```python
from build123d import *

# Parameters (mm, degrees)
SKETCH1_W           = 3
SKETCH1_H           = 7
BOSS_EXTRUDE1_DEPTH = 3


with BuildPart() as part:
    # Sketch1 → Boss-Extrude1 (new body)
    with BuildSketch(Plane(origin=(0, 0, 0), x_dir=(1, 0, 0), z_dir=(0, 1, 0))):
        Polygon((0, 35), (0, 28), (0, 21), (0, 14), (0, 7), (0, 0), (33, 0), (33, 7), (33, 14), (33, 21), (33, 28), (33, 35), (33, 42), (28.5, 42), (28.5, 39), (21.5, 39), (21.5, 42), (11.5, 42), (11.5, 39), (4.5, 39), (4.5, 42), (0, 42), align=None)
        with Locations((-1.5, 38.5)):
            Rectangle(SKETCH1_W, SKETCH1_H)
        with Locations((-1.5, 24.5)):
            Rectangle(SKETCH1_W, SKETCH1_H)
        with Locations((-1.5, 10.5)):
            Rectangle(SKETCH1_W, SKETCH1_H)
        with Locations((34.5, 10.5)):
            Rectangle(SKETCH1_W, SKETCH1_H)
        with Locations((34.5, 24.5)):
            Rectangle(SKETCH1_W, SKETCH1_H)
        with Locations((34.5, 38.5)):
            Rectangle(SKETCH1_W, SKETCH1_H)
        Polygon((33, 0), (0, 0), (-3, 0), (-3, -1.2), (36, -1.2), (36, 0), align=None)
    extrude(amount=BOSS_EXTRUDE1_DEPTH)


solid = part.part
```
Input: part model. Units: mm. Frame: model coordinates. A direction names the side the tool comes from. Round coordinates to 2 decimals unless told otherwise and drop trailing zeros. Loops run counter-clockwise (first coordinate to the right, second up) from the corner with the lowest first, then second, coordinate; pieces in that order, holes last. Notation, with made-up numbers: M -30,76 L 19,76 A16 cw 19,86 Z; hole C 62.5,80.5 d8. An arc over 180 degrees is marked long. Answer in a Markdown table with one row per item. Add a question column.
1. Section A-A (z = -31). Output: boundary loops of the cut face in (x, y), and give its area (3 significant figures).
2. Contact query for flat-ended pins moving along their axis: pin 1 (5 mm diameter, centred on x = 20, z = -10.5, fed in from -Y); pin 2 (1.5 mm diameter, centred on y = 1.5, z = -2, fed in from +X). Output: stop coordinate, or through.
3. Mould query, pull axis Z, two halves, no side actions, for faces 1 (the face through (16, 1, 1.2)), 2 (the face through (0, 1, -18)), 3 (the face through (28.5, 1, -41)). Classes: released by +Z, released by -Z, zero draft, split by the parting line, or undercut.
4. Set-up query: faces 4 (the face through (36, 1, -38)), 5 (the face through (34, 1, -7)), 6 (the face through (-2, 1, -7)), 7 (the face through (21.5, 1, -40)). Return all of +Z, -Z, +X, -X, +Y, -Y with unobstructed straight access to the full face (end or side cutting, diameter ignored); none if empty.
5. Ray query, probe 1 along Z at (x, y) = (34, 0.3); probe 2 along X at (y, z) = (0.6, -2.5); probe 3 along Z at (x, y) = (6.5, 0.4). Return the intervals inside material, ascending.
Values follow:
| question | item | result |
|---|---|---|
| 1 | outline | M 0,0 L 33,0 L 33,3 L 0,3 Z |
| 1 | area | 99.0 mm^2 |
| 2 | pin 1 | y = 0 |
| 2 | pin 2 | x = 33 |
| 3 | face 1 | released by +Z |
| 3 | face 2 | undercut |
| 3 | face 3 | zero draft |
| 4 | face 4 | +Z, -Z, +X, +Y, -Y |
| 4 | face 5 | +X, +Y, -Y |
| 4 | face 6 | -X, +Y, -Y |
| 4 | face 7 | -Z, +Y, -Y |
| 5 | probe 1 | -42 to -35, -28 to -21, -14 to -7, 0 to 1.2 |
| 5 | probe 2 | 0 to 33 |
| 5 | probe 3 | -39 to 1.2 |
